Verification items for the finished model (mm, model axes). A direction names the side the tool comes from. Coordinates: 2 decimals unless noted, no trailing zeros. Order: outer loops, then holes, each group sorted by start corner. A loop starts at its lowest first (then second) coordinate and runs counter-clockwise, first axis right, second up. Notation, with made-up numbers: M 63,11 L 91,11 A13 cw 91,31 Z; hole C 65,42.25 d9. An arc over 180 degrees is marked long. Return JSON: item names as keys, results as strings. Group by question number.
1. Material ranges on line 1 along Y through (x, z) = (-66.5, -4.6); line 2 along Y through (x, z) = (-78.5, -3.65); line 3 along X through (y, z) = (-19, -3.2), recorded low to high.
2. Section check C-C, the plane y = 33. Record the cut outline in (x, z), plus the area to 3 significant figures.
3. Section check B-B, the plane x = -69.25. Record the cut outline in (y, z), plus the area to 3 significant figures.
4. Mould release check, pull along X, two halves, no side actions. Record for faces 4 (the flat face through (-72.7, 47, -3)), 5 (the flat face through (-65.35, -38, -3)), 6 (the cylindrical face through (-76.7, -24.5, -3)), 7 (the flat face through (-76, -32.39, -3)): +X half, -X half, draft (parallel to the pull), parting line (faces both ways), or undercut.
5. Gauge pin test, flat ends, axial feed: pin 1 (3 mm diameter, centred on x = -70.5, z = -2.5, fed in from -Y); pin 2 (1.8 mm diameter, centred on y = -56, z = -2, fed in from +X); pin 3 (3 mm diameter, centred on x = -69, z = -2.5, fed in from +Y). Record the tip position at first contact, or that the pin passes through.
6. Set-up check for faces 1 (the flat face through (-72.089, -18, -3)), 2 (the flat face through (-69, -54.437, -3)), 3 (the flat face through (-72.7, -38, -3)): record each of +Z, -Z, +X, -X, +Y, -Y from which the full face is reachable in a straight line by a thin tool's end or side.
7. Section check A-A, the plane z = -4.3. Record the cut outline in (x, y).
8. Section check D-D, the plane x = -75. Record the cut outline in (y, z), plus the area to 3 significant figures.
```python
from build123d import *

# Parameters (mm, degrees)
SZKIC1_W                    = 14.1
SZKIC1_H                    = 136.58
DODANIE_WYCI_GNI_CIE1_DEPTH = 6
PRZENIE_CIAN_1_BY           = 6
SZKIC3_W                    = 6.75
SZKIC3_H                    = 10.4
SZKIC3_W_2                  = 6.95
SZKIC3_H_2                  = 6.4
SZKIC3_H_3                  = 6.342942851
WYTNIJ_WYCI_GNI_CIE1_DEPTH  = 107.058352026
SZKIC4_R                    = 1.55
WYTNIJ_WYCI_GNI_CIE2_DEPTH  = 107.058352026


with BuildPart() as part:
    # Szkic1 → Dodanie-wyciągnięcie1 (new body)
    with BuildSketch(Plane.XY):
        with Locations((-72.400450183, 1.710000001)):
            Rectangle(SZKIC1_W, SZKIC1_H)
    extrude(amount=-DODANIE_WYCI_GNI_CIE1_DEPTH)

    # Przenieś ścianę1: a face moved inward by 6.0
    extrude(part.faces().sort_by_distance((-72.400450183, -66.579999999, -3))[0], amount=PRZENIE_CIAN_1_BY, dir=(0, 1, 0), mode=Mode.SUBTRACT)

    # Szkic3 → Wytnij-wyciągnięcie1 (cut, through all)
    with BuildSketch(Plane.XY):
        with Locations((-76.075450183, 47.000000001)):
            Rectangle(SZKIC3_W, SZKIC3_H)
        with Locations((-76.075450183, -37.590311699)):
            Rectangle(SZKIC3_W, SZKIC3_H)
        with Locations((-68.613894602, 67.000000001)):
            Rectangle(SZKIC3_W_2, SZKIC3_H_2)
        with Locations((-68.613894602, 27.000000001)):
            Rectangle(SZKIC3_W_2, SZKIC3_H_2)
        with Locations((-68.625450183, -57.608528574)):
            Rectangle(SZKIC3_W_2, SZKIC3_H_3)
        with Locations((-68.613894602, -17.579999999)):
            Rectangle(SZKIC3_W_2, SZKIC3_H_2)
    extrude(amount=-WYTNIJ_WYCI_GNI_CIE1_DEPTH, mode=Mode.SUBTRACT)

    # Szkic4 → Wytnij-wyciągnięcie2 (cut, through all)
    with BuildSketch(Plane.XY):
        with Locations((-75.450450183, 61.000000001)):
            Circle(SZKIC4_R)
        with Locations((-75.450450183, -51.579999999)):
            Circle(SZKIC4_R)
        with Locations((-75.450450183, 33.000000001)):
            Circle(SZKIC4_R)
        with Locations((-75.450450183, -23.579999999)):
            Circle(SZKIC4_R)
    extrude(amount=-WYTNIJ_WYCI_GNI_CIE2_DEPTH, mode=Mode.SUBTRACT)


solid = part.part
```
Answers follow:
{
 "1": {"line 1": "-54.44 to -20.78, -14.38 to 23.8, 30.2 to 63.8", "line 2": "-60.58 to -42.79, -32.39 to 41.8, 52.2 to 70", "line 3": "-79.45 to -72.09"},
 "2": {"outline": "M -79.45,-6 L -77,-6 L -77,0 L -79.45,0 Z; M -73.9,-6 L -65.35,-6 L -65.35,0 L -73.9,0 Z", "area": "66.0 mm^2"},
 "3": {"outline": "M -54.44,-6 L -20.78,-6 L -20.78,0 L -54.44,0 Z; M -14.38,-6 L 23.8,-6 L 23.8,0 L -14.38,0 Z; M 30.2,-6 L 63.8,-6 L 63.8,0 L 30.2,0 Z", "area": "633 mm^2"},
 "4": {"face 4": "-X half", "face 5": "+X half", "face 6": "undercut", "face 7": "draft"},
 "5": {"pin 1": "y = -54.44", "pin 2": "x = -72.1", "pin 3": "y = 63.8"},
 "6": {"face 1": "+Z, -Z, +X", "face 2": "+Z, -Z, +X, -Y", "face 3": "+Z, -Z, -X"},
 "7": {"outline": "M -79.45,-60.58 L -72.1,-60.58 L -72.1,-54.44 L -65.35,-54.44 L -65.35,-20.78 L -72.09,-20.78 L -72.09,-14.38 L -65.35,-14.38 L -65.35,23.8 L -72.09,23.8 L -72.09,30.2 L -65.35,30.2 L -65.35,63.8 L -72.09,63.8 L -72.09,70 L -79.45,70 L -79.45,52.2 L -72.7,52.2 L -72.7,41.8 L -79.45,41.8 L -79.45,-32.39 L -72.7,-32.39 L -72.7,-42.79 L -79.45,-42.79 Z; hole C -75.45,-51.58 d3.1; hole C -75.45,-23.58 d3.1; hole C -75.45,33 d3.1; hole C -75.45,61 d3.1"},
 "8": {"outline": "M -60.58,-6 L -53.06,-6 L -53.06,0 L -60.58,0 Z; M -50.1,-6 L -42.79,-6 L -42.79,0 L -50.1,0 Z; M -32.39,-6 L -25.06,-6 L -25.06,0 L -32.39,0 Z; M -22.1,-6 L 31.52,-6 L 31.52,0 L -22.1,0 Z; M 34.48,-6 L 41.8,-6 L 41.8,0 L 34.48,0 Z; M 52.2,-6 L 59.52,-6 L 59.52,0 L 52.2,0 Z; M 62.48,-6 L 70,-6 L 70,0 L 62.48,0 Z", "area": "587 mm^2"}
}
